CAD build for the part. Positions are in the model's coordinates, mm. Round coordinates to 2 decimals unless told otherwise and drop trailing zeros. Order: outer loops, then holes, each group sorted by start corner. A loop starts at its lowest first (then second) coordinate and runs counter-clockwise, first axis right, second up. Notation, with made-up numbers: (59.25, 57.5) - (98.25, 57.5) arc R29 ccw to (98.25, 96.5) - close; hole circle Ø10 at (86, 1). An arc over 180 degrees is marked (long way). Use one line per item in the form item = value. Start each with the question number.
from build123d import *

# Parameters (mm, degrees)
F1_DEPTH = 38.1
F2_R     = 5.08
F3_R     = 5.08


with BuildPart() as f1:
    # F0 (on Front) → F1 (new body)
    with BuildSketch(Plane.XZ):
        Polygon((1288.923878, 939.480245), (135.55616, -189.862576), (171.830923, -278.764475), (1390.051439, 914.080245), (1390.051439, 939.480245), align=None)
    extrude(amount=F1_DEPTH)

    # F2
    f2_edges = [f1.edges().sort_by_distance(p)[0] for p in [
        (712.240019, -38.1, 374.808834),
        (712.240019, 0, 374.808834),
        (780.941181, -38.1, 317.657885),
    ]]
    fillet(f2_edges, radius=F2_R)

    # F3
    f3_edges = [f1.edges().sort_by_distance(p)[0] for p in [
        (780.941181, 0, 317.657885),
    ]]
    fillet(f3_edges, radius=F3_R)


solid = f1.part
(1) Slice it at A-A (y = -23.5). Give the cut face in (x, z).
(2) Wall check: line 1 (Z direction, x = 1173, y = -28.5); line 2 (Z direction, x = 724, y = -13.5); line 3 (X direction, y = -5.5, z = -196). Give the ranges that are in metal, low to high. Write a range as [from, to].
(3) Flat gauge pins, fed straight in: P1, Ø1, axis at x = 553, y = -10, coming from the -Z side; P2, Ø3, axis at y = -32, z = 778.5, coming from the +X side; P3, Ø4, axis at x = 1093, y = -27.5, coming from the -Z side. Where does each tip first touch, or does it go through?
Results list:
q1.outline = (135.56, -189.86) - (171.83, -278.76) - (1390.05, 914.08) - (1390.05, 939.48) - (1288.92, 939.48) - close
q2.line_1 = [701.55, 825.97]
q2.line_2 = [261.9, 386.32]
q2.line_3 = [138.06, 256.36]
q3.P1 = 93.98
q3.P2 = 1253.12
q3.P3 = 621.26
